Here's how the part is built. I have some questions about the finished solid (model axes, mm). A direction names the side the tool comes from. Round coordinates to 2 decimals unless told otherwise and drop trailing zeros. Write each loop counter-clockwise with the first axis right and the second up, starting at its lowest first coordinate (ties: lowest second). Pieces come first, ordered by that corner, then holes. Notation, with made-up numbers: (89, -39.5) -> (117, -39.5) arc R22 cw to (117, -23.5) -> close; hole circle Ø4 at (73, -6). An arc over 180 degrees is marked (long way). Put each result on its own line as item: value. Start each with the question number.
1. For pin 1 (8 mm diameter, centred on x = -10, y = -15, fed in from -Z); pin 2 (6 mm diameter, centred on y = 3.5, z = -45.5, fed in from +X); pin 3 (2.5 mm diameter, centred on x = 3, z = 29.5, fed in from +Y), each with a flat end and sliding along its axis, tell me the tip position at first contact or that it passes through.
2. We'd pull the mould along Z, two halves only. Please class faces 1 (the face through (-27.643, 0, 0)), 2 (the face through (-22.072, 0.055, -1.257)): +Z half, -Z half, draft (parallel to the pull), parting line (faces both ways), or undercut.
3. Suppose I cut it at B-B (x = -15). Please give me the cut outline in (y, z).
4. Suppose I cut it at A-A (z = 0). Please give me the cut outline in (x, y), then the cut area to 3 significant figures.
5. Suppose I cut it at C-C (y = -13). Please give me the cut outline in (x, z).
6. Which directions (+Z, -Z, +X, -X, +Y, -Y) give clear straight access to the entire face, cutting with the end or side of a thin tool? Please do faces 3 (the face through (-4, -7.112, 29)), 4 (the face through (27.46, -1.226, 0.638)), 5 (the face through (-0.42, -17.96, 25.7)).
7. Suppose I cut it at D-D (y = 0). Please give me the cut outline in (x, z).
8. I need wall thicknesses on probe 1 along Z at (x, y) = (-14, -1.5); probe 2 along Z at (x, y) = (-6, -12); probe 3 along Z at (x, y) = (16, -10.5). Which ranges of each line are inside material? Lowest first, please. Write a range as from..to.
```python
from build123d import *

# Parameters (mm, degrees)
F6_DEPTH = 3.302
F7_W     = 13.8215459883
F7_H     = 1.2585521908
F7_W_2   = 37.9781834781
F7_H_2   = 1.381920767


with BuildPart() as f1:
    # F0 (on Front) → F1 (revolve)
    with BuildSketch(Plane.XZ):
        with BuildLine():
            ThreePointArc((0, 36.5393093155), (-11.4251104851, 28.3988603898), (-7.4618768804, 14.9417864989))
            ThreePointArc((-7.4618768804, 14.9417864989), (-16.356873737, 3.3747995359), (-12.7664426916, -10.7682185787))
            ThreePointArc((-12.7664426916, -10.7682185787), (-24.1091703633, -38.8838765875), (0, -57.2658133922))
            Line((0, -57.2658133922), (0, 36.5393093155))
        make_face()
    revolve(axis=Axis((0, 0, -10.3632520383), (0, 0, -1)))

    # F2 (on Right) → F3 (revolve)
    with BuildSketch(Plane.YZ):
        Polygon((-24.0200255066, 24.3646577001), (-11.4886462688, 24.3646577001), (-11.3669829443, 27.2845905274), align=None)
    revolve(axis=Axis((0, -17.7543358877, 24.3646577001), (0, -1, 0)))

    # F5 (on offset) → F6 (cut)
    with BuildSketch(Plane.XZ.offset(10.414)):
        with BuildLine():
            add(Edge.make_bspline(
                [(-5.6940768845, 30.6755248457), (-6.4590711966, 29.4584885127), (-2.8828964047, 28.0595520455), (0.6932783872, 26.6606155783), (-2.1179020926, 29.2765883785), (-4.9290825725, 31.8925611787), (-5.6940768845, 30.6755248457)],
                knots=[0, 0, 0, 2.0943951024, 2.0943951024, 4.1887902048, 4.1887902048, 6.2831853072, 6.2831853072, 6.2831853072], degree=2, weights=[1, 0.5, 1, 0.5, 1, 0.5, 1]))
        make_face()
        with BuildLine():
            add(Edge.make_bspline(
                [(5.3165038116, 30.7971872389), (2.1750298927, 33.0720474057), (1.8295611088, 29.2884281393), (1.484092325, 25.5048088729), (4.9710350278, 27.0135679726), (8.4579777306, 28.5223270722), (5.3165038116, 30.7971872389)],
                knots=[4.7123889804, 4.7123889804, 4.7123889804, 6.8067840828, 6.8067840828, 8.9011791852, 8.9011791852, 10.9955742876, 10.9955742876, 10.9955742876], degree=2, weights=[1, 0.5, 1, 0.5, 1, 0.5, 1]))
        make_face()
    extrude(amount=-F6_DEPTH, mode=Mode.SUBTRACT)

    # F7 (on Front) → F8 (revolve)
    with BuildSketch(Plane.XZ):
        with Locations((-20.7323189825, 0.6292760954)):
            Rectangle(F7_W, F7_H)
        with Locations((18.9890917391, 0.6909603835)):
            Rectangle(F7_W_2, F7_H_2)
    revolve(axis=Axis((-13.8215459883, 0, 0), (-1, 0, 0)))


solid = f1.part
```
Verdict:
1. pin 1: stops at z = -52.96
1. pin 2: stops at x = 22.6
1. pin 3: stops at y = 11.17
2. face 1: draft
2. face 2: undercut
3. outline: circle Ø40 at (0, -32.26); circle Ø14.69 at (0, 0)
4. outline: (-27.64, -1.26) -> (-16.65, -1.26) arc R16.7 ccw to (16.64, -1.38) -> (37.98, -1.38) -> (37.98, 1.38) -> (16.64, 1.38) arc R16.7 ccw to (-16.65, 1.26) -> (-27.64, 1.26) -> close
4. area: 963 mm^2
5. outline: circle Ø42.71 at (0, -32.26); circle Ø20.97 at (0, 0); circle Ø5.09 at (0, 24.36)
6. face 3: none
6. face 4: +X
6. face 5: -Y
7. outline: (-27.64, -1.26) -> (-16.65, -1.26) arc R16.7 ccw to (-12.77, -10.77) arc R25 ccw (long way) to (12.77, -10.77) arc R16.7 ccw to (16.64, -1.38) -> (37.98, -1.38) -> (37.98, 1.38) -> (16.64, 1.38) arc R16.7 ccw to (7.46, 14.94) arc R12.09 ccw (long way) to (-7.46, 14.94) arc R16.7 ccw to (-16.65, 1.26) -> (-27.64, 1.26) -> close
8. probe 1: z = -52.92..-11.6, -8.98..8.98
8. probe 2: z = -53.36..-11.17, -9.95..9.95
8. probe 3: z = -48.35..-16.18
